Verification items for the finished model (mm, model axes). Round coordinates to 2 decimals unless told otherwise and drop trailing zeros. Order: outer loops, then holes, each group sorted by start corner. A loop starts at its lowest first (then second) coordinate and runs counter-clockwise, first axis right, second up.
```python
from build123d import *

# Parameters (mm, degrees)
CIRPATTERN1_COUNT = 2
CIRPATTERN1_ANGLE = 116.565051177


with BuildPart() as part:
    # Sketch1 → Revolve1 (revolve)
    with BuildSketch(Plane(origin=(0, 0, 0), x_dir=(1, 0, 0), z_dir=(0, 1, 0))):
        with BuildLine():
            Line((0, -100), (0, 100))
            ThreePointArc((0, 100), (100, 0), (0, -100))
        make_face()
    revolve(axis=Axis((0, 0, 100), (0, 0, -1)))

    # Sketch2 → Cut-Revolve1 (revolve, cut)
    with BuildSketch(Plane.XY):
        with BuildLine():
            Line((0, 245.843235607), (0, 36.168568135))
            ThreePointArc((0, 36.168568135), (-104.837333736, 141.005901871), (0, 245.843235607))
        make_face()
    cut_revolve1 = revolve(axis=Axis((0, 245.843235607, 0), (0, -1, 0)), mode=Mode.SUBTRACT)

    # Mirror1: Cut-Revolve1 across plane
    add(cut_revolve1.mirror(Plane.ZX), mode=Mode.SUBTRACT)

    # CirPattern1: Cut-Revolve1 ×2 about axis
    cirpattern1_axis = Axis((0, 0, 0), (0, 0, 1))
    for i in range(1, CIRPATTERN1_COUNT):
        add(cut_revolve1.rotate(cirpattern1_axis, i * CIRPATTERN1_ANGLE / (CIRPATTERN1_COUNT - 1)), mode=Mode.SUBTRACT)

    # CirPattern1 copy 1 sketch → CirPattern1 copy 1 (revolve, cut)
    with BuildSketch(Plane(origin=(0, 0, 0), x_dir=(-0.44721359549996187, 0.8944271909999139, 0), z_dir=(0, 0, 1))):
        with BuildLine():
            Line((0, -245.843235607), (0, -36.168568135))
            ThreePointArc((0, -36.168568135), (-104.837333736, -141.005901871), (0, -245.843235607))
        make_face()
    revolve(axis=Axis((219.888874651, 109.944437325, 0), (0.894427190999914, 0.4472135954999616, 0)), mode=Mode.SUBTRACT)

    # CirPattern2 copy 1 sketch → CirPattern2 copy 1 (revolve, cut)
    with BuildSketch(Plane(origin=(0, 0, 0), x_dir=(-0.13819660112501175, 0.8944271909999139, 0.42532540417602366), z_dir=(0.9510565162951535, 0, 0.30901699437494745))):
        with BuildLine():
            Line((0, 245.843235607), (0, 36.168568135))
            ThreePointArc((0, 36.168568135), (-104.837333736, 141.005901871), (0, 245.843235607))
        make_face()
    revolve(axis=Axis((-67.949399141, -109.944437325, 209.126747097), (0.2763932022500204, 0.44721359549996215, -0.8506508083520379)), mode=Mode.SUBTRACT)

    # CirPattern2 copy 2 sketch → CirPattern2 copy 2 (revolve, cut)
    with BuildSketch(Plane(origin=(0, 0, 0), x_dir=(0.36180339887499263, 0.8944271909999139, 0.2628655560595692), z_dir=(0.5877852522924732, 0, -0.8090169943749473))):
        with BuildLine():
            Line((0, 245.843235607), (0, 36.168568135))
            ThreePointArc((0, 36.168568135), (-104.837333736, 141.005901871), (0, 245.843235607))
        make_face()
    revolve(axis=Axis((177.893836466, -109.944437325, 129.247437663), (-0.7236067977499772, 0.44721359549996215, -0.5257311121191324)), mode=Mode.SUBTRACT)

    # CirPattern2 copy 3 sketch → CirPattern2 copy 3 (revolve, cut)
    with BuildSketch(Plane(origin=(0, 0, 0), x_dir=(0.36180339887499274, 0.8944271909999137, -0.26286555605956907), z_dir=(-0.587785252292473, 0, -0.8090169943749476))):
        with BuildLine():
            Line((0, 245.843235607), (0, 36.168568135))
            ThreePointArc((0, 36.168568135), (-104.837333736, 141.005901871), (0, 245.843235607))
        make_face()
    revolve(axis=Axis((177.893836466, -109.944437325, -129.247437663), (-0.7236067977499774, 0.4472135954999621, 0.5257311121191323)), mode=Mode.SUBTRACT)

    # CirPattern2 copy 4 sketch → CirPattern2 copy 4 (revolve, cut)
    with BuildSketch(Plane(origin=(0, 0, 0), x_dir=(-0.13819660112501164, 0.8944271909999139, -0.4253254041760237), z_dir=(-0.9510565162951536, 0, 0.30901699437494723))):
        with BuildLine():
            Line((0, 245.843235607), (0, 36.168568135))
            ThreePointArc((0, 36.168568135), (-104.837333736, 141.005901871), (0, 245.843235607))
        make_face()
    revolve(axis=Axis((-67.949399141, -109.944437325, -209.126747097), (0.2763932022500202, 0.44721359549996215, 0.850650808352038)), mode=Mode.SUBTRACT)

    # CirPattern2 copy 5 sketch → CirPattern2 copy 5 (revolve, cut)
    with BuildSketch(Plane(origin=(0, 0, 0), x_dir=(-0.13819660112501175, 0.8944271909999139, 0.42532540417602366), z_dir=(0.9510565162951535, 0, 0.30901699437494745))):
        with BuildLine():
            Line((0, -245.843235607), (0, -36.168568135))
            ThreePointArc((0, -36.168568135), (-104.837333736, -141.005901871), (0, -245.843235607))
        make_face()
    revolve(axis=Axis((67.949399141, 109.944437325, -209.126747097), (0.2763932022500205, 0.4472135954999616, -0.8506508083520381)), mode=Mode.SUBTRACT)

    # CirPattern2 copy 6 sketch → CirPattern2 copy 6 (revolve, cut)
    with BuildSketch(Plane(origin=(0, 0, 0), x_dir=(0.36180339887499263, 0.8944271909999139, 0.2628655560595692), z_dir=(0.5877852522924732, 0, -0.8090169943749473))):
        with BuildLine():
            Line((0, -245.843235607), (0, -36.168568135))
            ThreePointArc((0, -36.168568135), (-104.837333736, -141.005901871), (0, -245.843235607))
        make_face()
    revolve(axis=Axis((-177.893836466, 109.944437325, -129.247437663), (-0.7236067977499774, 0.4472135954999616, -0.5257311121191326)), mode=Mode.SUBTRACT)

    # CirPattern2 copy 7 sketch → CirPattern2 copy 7 (revolve, cut)
    with BuildSketch(Plane(origin=(0, 0, 0), x_dir=(0.36180339887499274, 0.8944271909999137, -0.26286555605956907), z_dir=(-0.587785252292473, 0, -0.8090169943749476))):
        with BuildLine():
            Line((0, -245.843235607), (0, -36.168568135))
            ThreePointArc((0, -36.168568135), (-104.837333736, -141.005901871), (0, -245.843235607))
        make_face()
    revolve(axis=Axis((-177.893836466, 109.944437325, 129.247437663), (-0.7236067977499776, 0.44721359549996154, 0.5257311121191325)), mode=Mode.SUBTRACT)

    # CirPattern2 copy 8 sketch → CirPattern2 copy 8 (revolve, cut)
    with BuildSketch(Plane(origin=(0, 0, 0), x_dir=(-0.13819660112501164, 0.8944271909999139, -0.4253254041760237), z_dir=(-0.9510565162951536, 0, 0.30901699437494723))):
        with BuildLine():
            Line((0, -245.843235607), (0, -36.168568135))
            ThreePointArc((0, -36.168568135), (-104.837333736, -141.005901871), (0, -245.843235607))
        make_face()
    revolve(axis=Axis((67.949399141, 109.944437325, 209.126747097), (0.2763932022500203, 0.4472135954999616, 0.8506508083520382)), mode=Mode.SUBTRACT)

    # CirPattern2 copy 9 sketch → CirPattern2 copy 9 (revolve, cut)
    with BuildSketch(Plane(origin=(0, 0, 0), x_dir=(0.30901699437494745, 0, -0.9510565162951535), z_dir=(0.9510565162951535, 0, 0.30901699437494745))):
        with BuildLine():
            Line((0, 245.843235607), (0, 36.168568135))
            ThreePointArc((0, 36.168568135), (-104.837333736, 141.005901871), (0, 245.843235607))
        make_face()
    revolve(axis=Axis((0, 245.843235607, 0), (0, -1, 0)), mode=Mode.SUBTRACT)

    # CirPattern2 copy 10 sketch → CirPattern2 copy 10 (revolve, cut)
    with BuildSketch(Plane(origin=(0, 0, 0), x_dir=(-0.8090169943749473, 0, -0.5877852522924732), z_dir=(0.5877852522924732, 0, -0.8090169943749473))):
        with BuildLine():
            Line((0, 245.843235607), (0, 36.168568135))
            ThreePointArc((0, 36.168568135), (-104.837333736, 141.005901871), (0, 245.843235607))
        make_face()
    revolve(axis=Axis((0, 245.843235607, 0), (0, -1, 0)), mode=Mode.SUBTRACT)

    # CirPattern2 copy 11 sketch → CirPattern2 copy 11 (revolve, cut)
    with BuildSketch(Plane(origin=(0, 0, 0), x_dir=(-0.8090169943749476, 0, 0.587785252292473), z_dir=(-0.587785252292473, 0, -0.8090169943749476))):
        with BuildLine():
            Line((0, 245.843235607), (0, 36.168568135))
            ThreePointArc((0, 36.168568135), (-104.837333736, 141.005901871), (0, 245.843235607))
        make_face()
    revolve(axis=Axis((0, 245.843235607, 0), (0, -1, 0)), mode=Mode.SUBTRACT)

    # CirPattern2 copy 12 sketch → CirPattern2 copy 12 (revolve, cut)
    with BuildSketch(Plane(origin=(0, 0, 0), x_dir=(0.30901699437494723, 0, 0.9510565162951536), z_dir=(-0.9510565162951536, 0, 0.30901699437494723))):
        with BuildLine():
            Line((0, 245.843235607), (0, 36.168568135))
            ThreePointArc((0, 36.168568135), (-104.837333736, 141.005901871), (0, 245.843235607))
        make_face()
    revolve(axis=Axis((0, 245.843235607, 0), (0, -1, 0)), mode=Mode.SUBTRACT)


solid = part.part
```
1) Sectioned sample at A-A on z = 24.5. Record the cut outline in (x, y).
2) Go/stop test with flat-tipped pins: pin 1 Ø8 at (x, y) = (16, 14.5) entering from -Z; pin 2 Ø4 at (y, z) = (-13, 29.5) entering from +X; pin 3 Ø2 at (x, z) = (18.5, 28.5) entering from +Y. Record where each tip stops, or that it passes through.
3) Sectioned sample at D-D on z = -3.5. Record the cut outline in (x, y), then the cut area to 3 significant figures.
4) Sectioned sample at B-B on y = -8. Record the cut outline in (x, z).
5) Sectioned sample at C-C on x = 13. Record the cut outline in (y, z), then the cut area to 3 significant figures.
6) Scan lines: probe 1 along X at (y, z) = (19, 1); probe 2 along Y at (x, z) = (-20, -11); probe 3 along Y at (x, z) = (-43.5, 13.5). Record each from-to range of solid material in increasing order.
Returned:
1. outline: (-41.31, -6.51) arc R101.93 cw to (-33.72, -20.01) arc R43.37 cw to (-2.82, -39.11) arc R101.93 cw to (12.65, -39.86) arc R92.35 cw to (41.31, 6.51) arc R101.93 cw to (33.72, 20.01) arc R43.37 cw to (2.82, 39.11) arc R101.93 cw to (-12.65, 39.86) arc R92.35 cw to start
2. pin 1: stops at z = -32.43
2. pin 2: stops at x = 23.16
2. pin 3: stops at y = 18.11
3. outline: (-48.37, 7.18) arc R104.78 cw to (-24.13, -39.04) arc R104.78 cw to (28.05, -40.05) arc R77.47 cw to (48.37, -7.18) arc R104.78 cw to (24.13, 39.04) arc R104.78 cw to (-28.05, 40.05) arc R77.47 cw to start
3. area: 5,270 mm2
4. outline: (-41.07, -26.96) arc R77.08 cw to (-38.33, -30.73) arc R89.21 cw to (12.94, -47.39) arc R77.08 cw to (17.39, -45.95) arc R89.21 cw to (49.07, -2.33) arc R77.08 cw to (49.07, 2.33) arc R89.21 cw to (17.39, 45.95) arc R77.08 cw to (12.94, 47.39) arc R89.21 cw to (-38.33, 30.73) arc R77.08 cw to (-41.07, 26.96) arc R89.21 cw to start
5. outline: (-39.76, -23.92) arc R55.35 cw to (-19.47, -40.01) arc R91.05 cw to (-8.03, -47.41) arc R101.57 cw to (39.17, -21.23) arc R104.03 cw to (39.17, 21.23) arc R101.57 cw to (-8.03, 47.41) arc R91.05 cw to (-19.47, 40.01) arc R55.35 cw to (-39.76, 23.92) arc R104.03 cw to start
5. area: 5,060 mm2
6. probe 1: x = -41.19 to 31
6. probe 2: y = -38.68 to 38.68
6. probe 3: y = 0.05 to 0.7
